Model file for the job. Use its own axes, mm. A direction names the side the tool comes from. Give positions to 0.01 mm unless a question says otherwise; leave off trailing zeros. Order: outer loops, then holes, each group sorted by start corner. A loop starts at its lowest first (then second) coordinate and runs counter-clockwise, first axis right, second up. Notation, with made-up numbers: M 86.5,49 L 124.5,49 A18 cw 124.5,74 Z; hole C -24.75,-5 d7. An arc over 180 degrees is marked long. Return JSON: item names as keys, results as strings. Group by question number.
1. 3-axis set-ups, long thin cutter, end or side, ignore diameter. For faces 4 (the face through (3.175, 31, 3)), 5 (the face through (7.62, 102, 3)): which of +Z, -Z, +X, -X, +Y, -Y reach the whole face in a straight line?
2. Slice it at C-C on z = 2.5. List the corners of the cut face in (x, y) (3 decimals), then the cut area to 3 significant figures.
3. Slice it at A-A on y = 77. List the corners of the cut face in (x, z) (3 decimals), then the cut area to 3 significant figures.
4. Two-plate mould, pull along Y, no slides. Class faces 1 (the face through (-0.07, 46.456, 3.131)), 2 (the face through (3.5, 101.7, 6.35)), 3 (the face through (-3.175, 30, 3)): released by +Y, released by -Y, zero draft, split by the parting line, or undercut.
5. Wall check: probe 1 along X at (y, z) = (124.5, 3.5); probe 2 along Y at (x, z) = (-3.5, 2); probe 3 along Y at (x, z) = (-3.25, 0.5) (3 decimals). Give the ranges that are in metal, low to high. Write a range as [from, to].
6. Slice it at B-B on x = 0. Give the number of separate pieces and of enclosed holes in the cut face, then the cut area to 3 significant figures.
7. Pin check, flat tips, straight feed: pin 1 (1.5 mm diameter, centred on x = 6, z = 3, fed in from +Y); pin 2 (2 mm diameter, centred on x = -2, y = 125, fed in from +Z); pin 3 (3 mm diameter, centred on x = 3, z = 3.5, fed in from +Y). Stop position of each tip, or through.
from build123d import *

# Parameters (mm, degrees)
SKETCH_2_R             = 3.96748
EXTRUDE_1_DEPTH        = 6.35
F_10_24_TAPPED_HOLE1_D = 3.7973


with BuildPart() as part:
    # 草图2 → 凸台-拉伸1 (new body)
    with BuildSketch(Plane.XY):
        with BuildLine():
            Line((-7.62, 0), (-7.62, 200.3806))
            ThreePointArc((-7.62, 200.3806), (0, 208.0006), (7.62, 200.3806))
            Line((7.62, 200.3806), (7.62, 0))
            ThreePointArc((7.62, 0), (0, -7.62), (-7.62, 0))
        make_face()
        with Locations((0, 200.3806)):
            Circle(SKETCH_2_R, mode=Mode.SUBTRACT)
        with BuildLine():
            Line((3.175, 185.5216), (3.175, 160.1216))
            ThreePointArc((3.175, 160.1216), (0, 156.9466), (-3.175, 160.1216))
            Line((-3.175, 160.1216), (-3.175, 185.5216))
            ThreePointArc((-3.175, 185.5216), (0, 188.6966), (3.175, 185.5216))
        make_face(mode=Mode.SUBTRACT)
        with BuildLine():
            Line((3.175, 149.9616), (3.175, 124.5616))
            ThreePointArc((3.175, 124.5616), (0, 121.3866), (-3.175, 124.5616))
            Line((-3.175, 124.5616), (-3.175, 149.9616))
            ThreePointArc((-3.175, 149.9616), (0, 153.1366), (3.175, 149.9616))
        make_face(mode=Mode.SUBTRACT)
        with BuildLine():
            Line((3.175, 114.4016), (3.175, 89.0016))
            ThreePointArc((3.175, 89.0016), (0, 85.8266), (-3.175, 89.0016))
            Line((-3.175, 89.0016), (-3.175, 114.4016))
            ThreePointArc((-3.175, 114.4016), (0, 117.5766), (3.175, 114.4016))
        make_face(mode=Mode.SUBTRACT)
        with BuildLine():
            Line((3.175, 78.8416), (3.175, 53.4416))
            ThreePointArc((3.175, 53.4416), (0, 50.2666), (-3.175, 53.4416))
            Line((-3.175, 53.4416), (-3.175, 78.8416))
            ThreePointArc((-3.175, 78.8416), (0, 82.0166), (3.175, 78.8416))
        make_face(mode=Mode.SUBTRACT)
        with BuildLine():
            Line((3.175, 43.2816), (3.175, 17.8816))
            ThreePointArc((3.175, 17.8816), (0, 14.7066), (-3.175, 17.8816))
            Line((-3.175, 17.8816), (-3.175, 43.2816))
            ThreePointArc((-3.175, 43.2816), (0, 46.4566), (3.175, 43.2816))
        make_face(mode=Mode.SUBTRACT)
    extrude(amount=EXTRUDE_1_DEPTH)

    # #10-24 Tapped Hole1 (through all)
    with Locations(Plane.XY.offset(6.35)):
        with Locations((0, 0)):
            Hole(F_10_24_TAPPED_HOLE1_D / 2)


solid = part.part
Result:
{
 "1": {"face 4": "+Z, -Z", "face 5": "+Z, -Z, +X, +Y, -Y"},
 "2": {"outline": "M -7.62,0 A7.62 ccw 7.62,0 L 7.62,200.381 A7.62 ccw -7.62,200.381 Z; hole C 0,200.381 d7.935; hole M -3.175,17.882 A3.175 ccw 3.175,17.882 L 3.175,43.282 A3.175 ccw -3.175,43.282 Z; hole M -3.175,53.442 A3.175 ccw 3.175,53.442 L 3.175,78.842 A3.175 ccw -3.175,78.842 Z; hole M -3.175,89.002 A3.175 ccw 3.175,89.002 L 3.175,114.402 A3.175 ccw -3.175,114.402 Z; hole M -3.175,124.562 A3.175 ccw 3.175,124.562 L 3.175,149.962 A3.175 ccw -3.175,149.962 Z; hole M -3.175,160.122 A3.175 ccw 3.175,160.122 L 3.175,185.522 A3.175 ccw -3.175,185.522 Z; hole C 0,0 d3.797", "area": "2,210 mm2"},
 "3": {"outline": "M -7.62,0 L -3.175,0 L -3.175,6.35 L -7.62,6.35 Z; M 3.175,0 L 7.62,0 L 7.62,6.35 L 3.175,6.35 Z", "area": "56.5 mm2"},
 "4": {"face 1": "undercut", "face 2": "zero draft", "face 3": "undercut"},
 "5": {"probe 1": "x = [-7.62, -3.17], [3.17, 7.62]", "probe 2": "y = [-6.77, 198.51], [202.25, 207.15]", "probe 3": "y = [-6.892, 198.105], [202.656, 207.273]"},
 "6": {"separate pieces": "8", "enclosed holes": "0", "area": "287 mm2"},
 "7": {"pin 1": "stops at y = 205.9", "pin 2": "passes through", "pin 3": "stops at y = 207.85"}
}
